Answer from the drawing. Dimensions are ordinates in mm from the lowest x, y and z of the part. Give positions to 0.01 mm unless a question says otherwise; leave off trailing zeros. Order: outer loops, then holes, each group sorted by start corner. A loop starts at its lowest first (then second) coordinate and runs counter-clockwise, first axis right, second up. Notation, with made-up numbers: (83.5, 16) -> (104.5, 16) arc R13 ccw to (104.5, 22) -> close; hole circle Ø2 at (71.25, 73.5). An arc over 180 degrees is marked (long way). One line per question, with ' | ' between items. Start each with the question number.
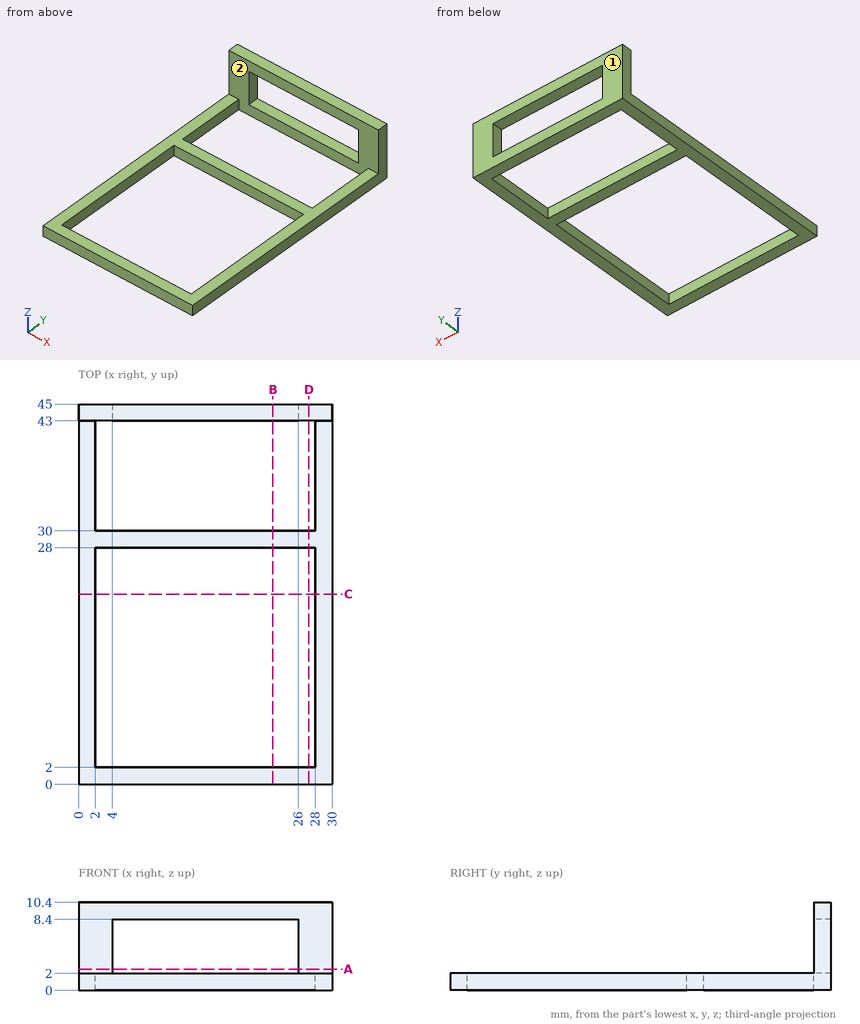
(1) The part is cut by section D-D on x = 27.25. Determine the outline of the cut face in (y, z).
(2) Determine the mould class of the marked faces 1 and 2 for opening direction X: pulls with the +X half, pulls with the -X half, needs draft (parallel to the pull), parting line crosses it, or undercut.
(3) The part is cut by section A-A on z = 2.5. Determine the outline of the cut face in (x, y).
(4) Consider line 1 (X direction, y = 16.5, z = 0.5); line 2 (Y direction, x = 22.5, z = 9); line 3 (Z direction, x = 1.75, y = 4.5). Determine where each line is inside the solid, lowest interval first.
(5) The part is cut by section B-B on x = 23. Determine the outline of the cut face in (y, z), plus the area to 3 significant figures.
(6) The part is cut by section C-C on y = 22.5. Determine the outline of the cut face in (x, z).
Result sheet:
1) outline: (0, 0) -> (2, 0) -> (2, 2) -> (0, 2) -> close; (28, 0) -> (30, 0) -> (30, 2) -> (28, 2) -> close; (43, 0) -> (45, 0) -> (45, 10.4) -> (43, 10.4) -> close
2) face 1: needs draft | face 2: undercut
3) outline: (0, 43) -> (4, 43) -> (4, 45) -> (0, 45) -> close; (26, 43) -> (30, 43) -> (30, 45) -> (26, 45) -> close
4) line 1: x = 0 to 2, 28 to 30 | line 2: y = 43 to 45 | line 3: z = 0 to 2
5) outline: (0, 0) -> (2, 0) -> (2, 2) -> (0, 2) -> close; (28, 0) -> (30, 0) -> (30, 2) -> (28, 2) -> close; (43, 0) -> (45, 0) -> (45, 2) -> (43, 2) -> close; (43, 8.4) -> (45, 8.4) -> (45, 10.4) -> (43, 10.4) -> close | area: 16.0 mm^2
6) outline: (0, 0) -> (2, 0) -> (2, 2) -> (0, 2) -> close; (28, 0) -> (30, 0) -> (30, 2) -> (28, 2) -> close
